from build123d import *

# Parameters (mm, degrees)
SKETCH_1_R          = 30
EXTRUDE_1_DEPTH     = 45
SKETCH_3_R          = 33.5
EXTRUDE_2_DEPTH     = 10
CUT_EXTRUDE_1_DEPTH = 73.591321795
SKETCH_5_R          = 3
CUT_EXTRUDE_2_DEPTH = 18
CHAMFER_1_SIZE      = 0.5


with BuildPart() as part:
    # 草图1 → 凸台-拉伸1 (new body)
    with BuildSketch(Plane.XY):
        with Locations(Location((0, 0, 0), (0, 0, 180))):
            Circle(SKETCH_1_R)
    extrude(amount=EXTRUDE_1_DEPTH)

    # 草图3 → 凸台-拉伸2 (add)
    with BuildSketch(Plane.XY.offset(45)):
        Circle(SKETCH_3_R)
    extrude(amount=EXTRUDE_2_DEPTH)

    # 草图4 → 切除-拉伸1 (cut, through all)
    with BuildSketch(Plane.XY.offset(55)):
        with BuildLine():
            Line((-5, 18.33030278), (-5, 22))
            Line((-5, 22), (5, 22))
            Line((5, 22), (5, 18.33030278))
            ThreePointArc((5, 18.33030278), (0, -19), (-5, 18.33030278))
        make_face()
    extrude(amount=-CUT_EXTRUDE_1_DEPTH, mode=Mode.SUBTRACT)

    # 草图5 → 切除-拉伸2 (cut)
    with BuildSketch(Plane.XY):
        with Locations((-12.5, 21.650635095)):
            Circle(SKETCH_5_R)
        with Locations((12.5, 21.650635095)):
            Circle(SKETCH_5_R)
        with Locations((25, 0)):
            Circle(SKETCH_5_R)
        with Locations((12.5, -21.650635095)):
            Circle(SKETCH_5_R)
        with Locations((-12.5, -21.650635095)):
            Circle(SKETCH_5_R)
        with Locations((-25, 0)):
            Circle(SKETCH_5_R)
    extrude(amount=CUT_EXTRUDE_2_DEPTH, mode=Mode.SUBTRACT)

    # 倒角1
    chamfer_1_edges = [part.edges().sort_by_distance(p)[0] for p in [
        (0, -19, 0),
        (0, -19, 55),
        (30, 0, 0),
        (-33.5, 0, 45),
        (-33.5, 0, 55),
    ]]
    chamfer(chamfer_1_edges, length=CHAMFER_1_SIZE)


solid = part.part
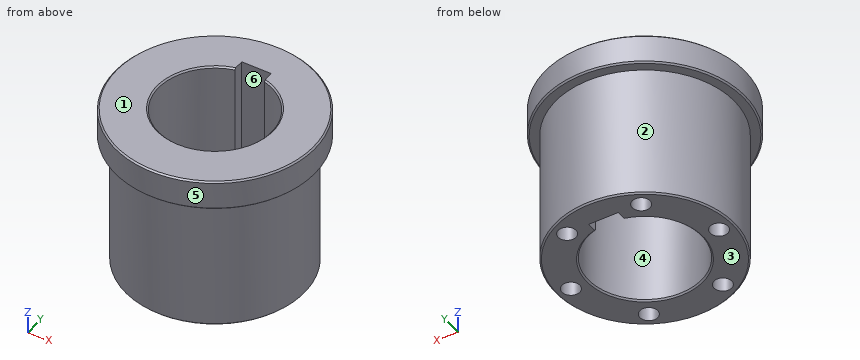
Geometry check sheet. Reference: the model listing, model coordinates, mm. Face numbers are marked on the shaded views. A direction names the side the tool comes from. Round coordinates to 2 decimals unless told otherwise and drop trailing zeros. Loops run counter-clockwise (first coordinate to the right, second up) from the corner with the lowest first, then second, coordinate; pieces in that order, holes last. Notation, with made-up numbers: (-30, 65.25) - (-4, 65.25) arc R25 ccw to (-4, 78.25) - close; hole circle Ø7 at (36.5, 43.25). An arc over 180 degrees is marked (long way). One line per question, with ' | ' between items. Start each with the question number.
1. Tool access check on the marked faces 1 and 2. Record the directions out of +Z, -Z, +X, -X, +Y, -Y that give a thin tool (end or side, any length) a straight path to the whole face; none if there is none.
2. Cross-section at A-A on x = 0. Record the cut outline in (y, z).
3. Draft check along Y on the marked faces 3, 4, 5 and 6. Enter one of: released by +Y, released by -Y, zero draft, split by the parting line, or undercut.
4. Cross-section at D-D on z = 16. Record the cut outline in (x, y), then the cut area to 3 significant figures.
5. Cross-section at B-B on z = 34. Record the cut outline in (x, y).
6. Depth check by flat-ended pin: pin 1 (2 mm diameter, centred on x = 2.5, z = 39, fed in from +Y); pin 2 (3 mm diameter, centred on x = 2, z = 32, fed in from -Y); pin 3 (1.5 mm diameter, centred on y = -22.5, z = 24, fed in from -X); pin 4 (1.5 mm diameter, centred on x = -16.5, y = 0, fed in from +Z). Enter the tip coordinate at first touch or a pass-through.
7. Scan lines: line 1 (Y direction, x = -10, z = 12); line 2 (X direction, y = -1.5, z = 10); line 3 (Y direction, x = -11.5, z = 31). Record each from-to range of solid material in increasing order. Write a range as [from, to].
Taken from the geometry:
1) face 1: +Z, +X, -X, +Y, -Y | face 2: -Z
2) outline: (-33.5, 45.5) - (-33, 45) - (-30, 45) - (-30, 0.5) - (-29.5, 0) - (-19.5, 0) - (-19, 0.5) - (-19, 54.5) - (-19.5, 55) - (-33, 55) - (-33.5, 54.5) - close; (22, 0) - (29.5, 0) - (30, 0.5) - (30, 45) - (33, 45) - (33.5, 45.5) - (33.5, 54.5) - (33, 55) - (22, 55) - close
3) face 3: zero draft | face 4: undercut | face 5: split by the parting line | face 6: undercut
4) outline: circle Ø60 at (0, 0); hole circle Ø6 at (-25, 0); hole circle Ø6 at (-12.5, -21.65); hole circle Ø6 at (-12.5, 21.65); hole (-5, 18.33) arc R19 ccw (long way) to (5, 18.33) - (5, 22) - (-5, 22) - close; hole circle Ø6 at (12.5, -21.65); hole circle Ø6 at (12.5, 21.65); hole circle Ø6 at (25, 0) | area: 1,490 mm²
5) outline: circle Ø60 at (0, 0); hole (-5, 18.33) arc R19 ccw (long way) to (5, 18.33) - (5, 22) - (-5, 22) - close
6) pin 1: y = 29.96 | pin 2: y = -30 | pin 3: x = -20.66 | pin 4: through
7) line 1: [-28.28, -23.31], [-19.99, -16.16], [16.16, 19.99], [23.31, 28.28] | line 2: [-29.96, -27.6], [-22.4, -18.94], [18.94, 22.4], [27.6, 29.96] | line 3: [-27.71, -15.12], [15.12, 27.71]
